CAD build for the part. Positions are in the model's coordinates, mm. A direction names the side the tool comes from. Give positions to 0.01 mm unless a question says otherwise; leave off trailing zeros. Write each loop counter-clockwise with the first axis right and the second up, starting at its lowest first coordinate (ties: lowest second). Pieces come first, ordered by that corner, then holes. Notation, with made-up numbers: (-11, 61) -> (2, 61) arc R17 cw to (2, 83) -> close; hole circle Ø8 at (3.25, 31). An arc over 180 degrees is marked (long way). Answer in a Markdown table with one row per item. Add a question column.
```python
from build123d import *

# Parameters (mm, degrees)
SKETCH_1_W          = 3
SKETCH_1_H          = 4
SKETCH_2_W          = 8.891252249
SKETCH_2_H          = 5
SKETCH_2_W_2        = 5
SKETCH_2_H_2        = 11.708042321
CUT_EXTRUDE_1_DEPTH = 5
EXTRUDE_1_REACH     = 29.911
SKETCH_3_W          = 7
SKETCH_3_H          = 7
SKETCH_4_W          = 5
SKETCH_4_H          = 7
CUT_EXTRUDE_2_DEPTH = 1.5
SKETCH_5_R          = 1.761378247
SKETCH_5_W          = 0.5
SKETCH_5_H          = 7
CUT_EXTRUDE_3_DEPTH = 11.9
SKETCH_6_R          = 1.396648932
EXTRUDE_2_DEPTH     = 1
SKETCH_7_R          = 0.55
CUT_EXTRUDE_4_DEPTH = 30.055980452
CHAMFER_1_SIZE      = 0.5
FILLET_1_R          = 0.1
CHAMFER_2_SIZE      = 0.1
FILLET_2_R          = 0.1
SKETCH_8_R          = 2
CUT_EXTRUDE_5_DEPTH = 5
CHAMFER_3_SIZE      = 0.5


with BuildPart() as part:
    # 草图1 → 旋转1 (revolve)
    with BuildSketch(Plane.XY, mode=Mode.PRIVATE) as revolve_1_sk:
        with Locations((1.5, 2)):
            Rectangle(SKETCH_1_W, SKETCH_1_H)
        Polygon((3, 0), (13, 0), (13, 5), (3, 5), (3, 4), align=None)
        Polygon((13, 0), (13, 5), (15, 0), align=None)
    revolve(revolve_1_sk.sketch.rotate(Axis((3, 0, 0), (1, 0, 0)), 90), axis=Axis((3, 0, 0), (1, 0, 0)))

    # 草图2 → 切除-拉伸1 (cut)
    with BuildSketch(Plane.ZY.offset(-6)):
        with Locations((6.945626125, 0)):
            Rectangle(SKETCH_2_W, SKETCH_2_H)
        with Locations((0, -8.354021161)):
            Rectangle(SKETCH_2_W_2, SKETCH_2_H_2)
        with Locations((0, 8.354021161)):
            Rectangle(SKETCH_2_W_2, SKETCH_2_H_2)
        with Locations((-6.945626125, 0)):
            Rectangle(SKETCH_2_W, SKETCH_2_H)
        Rectangle(SKETCH_2_W_2, SKETCH_2_H)
    extrude(amount=-CUT_EXTRUDE_1_DEPTH, mode=Mode.SUBTRACT)

    # 凸台-拉伸1: up to this cone (the profile starts outside it)
    extrude_1_end = Plane(origin=(27, 0, 0), z_dir=(-1, 0, 0)).offset(12.000001) * Cone(2.5e-06, 46.0275, 18.410999, align=(Align.CENTER, Align.CENTER, Align.MIN), mode=Mode.PRIVATE)
    # 草图3 → 凸台-拉伸1 (add, up to the surface)
    with BuildSketch(Plane.ZY.offset(-27), mode=Mode.PRIVATE) as extrude_1_sk1:
        Rectangle(SKETCH_3_W, SKETCH_3_H)
    extrude_1_tool1 = extrude(extrude_1_sk1.sketch, amount=EXTRUDE_1_REACH, mode=Mode.PRIVATE) - extrude_1_end
    add(extrude_1_tool1.solids().sort_by_distance((27, 0, 0))[0])

    # 草图4 → 切除-拉伸2 (cut)
    with BuildSketch(Plane(origin=(27, 0, 0), x_dir=(0, 0, -1), z_dir=(1, 0, 0))):
        Rectangle(SKETCH_4_W, SKETCH_4_H)
    extrude(amount=-CUT_EXTRUDE_2_DEPTH, mode=Mode.SUBTRACT)

    # 草图5 → 切除-拉伸3 (cut)
    with BuildSketch(Plane(origin=(25.5, 0, 0), x_dir=(0, 0, -1), z_dir=(1, 0, 0))):
        Circle(SKETCH_5_R)
        Rectangle(SKETCH_5_W, SKETCH_5_H)
    extrude(amount=-CUT_EXTRUDE_3_DEPTH, mode=Mode.SUBTRACT)

    # 草图6 → 凸台-拉伸2 (add)
    with BuildSketch(Plane.XY.offset(3.5)):
        with Locations(Location((21, 0, 0), (0, 0, 180))):
            Circle(SKETCH_6_R)
    extrude(amount=EXTRUDE_2_DEPTH)

    # 草图7 → 切除-拉伸4 (cut, through all)
    with BuildSketch(Plane.XY.offset(4.5)):
        with Locations((21, 0)):
            Circle(SKETCH_7_R)
    extrude(amount=-CUT_EXTRUDE_4_DEPTH, mode=Mode.SUBTRACT)

    # 倒角1
    chamfer_1_edges = [part.edges().sort_by_distance(p)[0] for p in [
        (20.45, 0, -3.5),
    ]]
    chamfer(chamfer_1_edges, length=CHAMFER_1_SIZE)

    # 圆角1
    fillet_1_edges = [part.edges().sort_by_distance(p)[0] for p in [
        (22.396648932, 0, 3.5),
    ]]
    fillet(fillet_1_edges, radius=FILLET_1_R)

    # 倒角2
    chamfer_2_edges = [part.edges().sort_by_distance(p)[0] for p in [
        (0, 0, -4),
        (3, 0, -5),
    ]]
    chamfer(chamfer_2_edges, length=CHAMFER_2_SIZE)

    # 圆角2
    fillet_2_edges = [part.edges().sort_by_distance(p)[0] for p in [
        (20.010050506, -3.5, -3.5),
        (20.010050506, 3.5, -3.5),
        (20.010050506, 3.5, 3.5),
        (20.010050506, -3.5, 3.5),
    ]]
    fillet(fillet_2_edges, radius=FILLET_2_R)

    # 草图8 → 切除-拉伸5 (cut)
    with BuildSketch(Plane.ZY):
        Circle(SKETCH_8_R)
    extrude(amount=-CUT_EXTRUDE_5_DEPTH, mode=Mode.SUBTRACT)

    # 倒角3
    chamfer_3_edges = [part.edges().sort_by_distance(p)[0] for p in [
        (0, 0, -2),
    ]]
    chamfer(chamfer_3_edges, length=CHAMFER_3_SIZE)


solid = part.part
```
Item 1: Drop flat-ended pins along their axis: pin 1 Ø1.1 at (y, z) = (-0.5, 1) entering from +X; pin 2 Ø0.9 at (x, z) = (9.5, -4) entering from +Y; pin 3 Ø1.6 at (x, y) = (26.5, -1) entering from +Z; pin 4 Ø0.7 at (x, y) = (21, 0) entering from +Z. Give the stop position or say it passes through.
Item 2: Slice it at B-B, the plane x = 21. State how many separate pieces and enclosed holes the cut face has, then the cut area to 3 significant figures.
Item 3: Slice it at A-A, the plane x = 18.25. List the corners of the cut face in (y, z).
Item 4: Which spindle directions (+Z, -Z, +X, -X, +Y, -Y) get a long thin tool onto all of the face, cutting with end or side? Do faces 1 (the face through (21, 1, 4.5)), 2 (the face through (13.6, 0, 0)), 3 (the face through (1.57, 3.905, -0.867)). Say none if no direction does.
Item 5: Probe L1, parallel to X at y = 0, z = 2.25; L2, parallel to Z at x = 21, y = 3; L3, parallel to X at y = -2.5, z = -1.75. List the from-to ranges inside material, lowest first. Write a range as from..to.
Item 6: Mould opens along Z. For faces 4 (the face through (20, 3, -0.25)), 5 (the face through (8, 3, -2.5)), 6 (the face through (19, 0, 3.5)), 7 (the face through (20, 3.5, -2)) say: released by +Z, released by -Z, zero draft, split by the parting line, or undercut.
Answer key:
| question | item | result |
|---|---|---|
| 1 | pin 1 | stops at x = 13.6 |
| 1 | pin 2 | stops at y = 3.52 |
| 1 | pin 3 | stops at z = 3.5 |
| 1 | pin 4 | passes through |
| 2 | separate pieces | 4 |
| 2 | enclosed holes | 0 |
| 2 | area | 35.1 mm² |
| 3 | outline | (-3.5, -3.4) arc R0.1 ccw to (-3.4, -3.5) -> (3.4, -3.5) arc R0.1 ccw to (3.5, -3.4) -> (3.5, -0.25) -> (1.74, -0.25) arc R1.76 cw to (-1.74, -0.25) -> (-3.5, -0.25) -> close; (-3.5, 0.25) -> (-1.74, 0.25) arc R1.76 cw to (1.74, 0.25) -> (3.5, 0.25) -> (3.5, 3.4) arc R0.1 ccw to (3.4, 3.5) -> (-3.4, 3.5) arc R0.1 ccw to (-3.5, 3.4) -> close |
| 4 | face 1 | +Z, +X, +Y, -Y |
| 4 | face 2 | +X |
| 4 | face 3 | -X |
| 5 | L1 | x = 0.25..6, 11..20.45, 21.55..25.5 |
| 5 | L2 | z = -3.5..-0.25, 0.25..3.5 |
| 5 | L3 | x = 0..6, 11..25.5 |
| 6 | face 4 | undercut |
| 6 | face 5 | undercut |
| 6 | face 6 | released by +Z |
| 6 | face 7 | zero draft |
